Geometry check sheet. Reference: the model listing, model coordinates, mm. A direction names the side the tool comes from. Coordinates: 2 decimals unless noted, no trailing zeros. Loops run counter-clockwise (first coordinate to the right, second up) from the corner with the lowest first, then second, coordinate; pieces in that order, holes last.
from build123d import *
from OCP.BRepFilletAPI import BRepFilletAPI_MakeChamfer

# Parameters (mm, degrees)
BOSS_EXTRUDE1_DEPTH     = 5
CHAMFER1_SIZE           = 5
CHAMFER1_SIZE2          = 18.660254038
CUT_EXTRUDE1_DEPTH      = 10
CUT_EXTRUDE1_DEPTH_BACK = 10


with BuildPart() as part:
    # Sketch1 → Boss-Extrude1 (new body)
    with BuildSketch(Plane(origin=(0, 0, 0), x_dir=(1, 0, 0), z_dir=(0, 1, 0))):
        Polygon((-7.5, 40), (7.5, 40), (7.5, -40), (1, -40), (1, -35), (-1, -35), (-1, -40), (-7.5, -40), align=None)
        with BuildLine():
            Line((-2.5, -25.078773429), (-2.5, 9.921226571))
            ThreePointArc((-2.5, 9.921226571), (0, 12.421226571), (2.5, 9.921226571))
            Line((2.5, 9.921226571), (2.5, -25.078773429))
            ThreePointArc((2.5, -25.078773429), (0, -27.578773429), (-2.5, -25.078773429))
        make_face(mode=Mode.SUBTRACT)
    extrude(amount=BOSS_EXTRUDE1_DEPTH)

    # Chamfer1: one chamfer whose edges measure the first distance from different faces: ONE call of the kernel's chamfer builder (chamfer() names one face for all edges)
    chamfer1_edges_1 = [part.edges().sort_by_distance(p)[0] for p in [
        (-7.5, 2.5, 40),
    ]]
    chamfer1_side_1 = [part.faces().sort_by_distance(p)[0] for p in [
        (-4.25, 2.5, 40),
    ]]
    chamfer1_edges_2 = [part.edges().sort_by_distance(p)[0] for p in [
        (7.5, 2.5, 40),
    ]]
    chamfer1_side_2 = [part.faces().sort_by_distance(p)[0] for p in [
        (4.25, 2.5, 40),
    ]]
    chamfer1 = BRepFilletAPI_MakeChamfer(part.part.solid().wrapped)
    for e in chamfer1_edges_1:
        chamfer1.Add(CHAMFER1_SIZE, CHAMFER1_SIZE2, e.wrapped, chamfer1_side_1[0].wrapped)  # the first distance lies on this face
    for e in chamfer1_edges_2:
        chamfer1.Add(CHAMFER1_SIZE, CHAMFER1_SIZE2, e.wrapped, chamfer1_side_2[0].wrapped)  # the first distance lies on this face
    add(Compound.cast(chamfer1.Shape()), mode=Mode.REPLACE)

    # Sketch2 → Cut-Extrude1 (cut, two sides: drawn at the far end of the back side and taken through both)
    with BuildSketch(Plane(origin=(0, 0, 0), x_dir=(0, 0, -1), z_dir=(1, 0, 0)).offset(-CUT_EXTRUDE1_DEPTH_BACK)):
        Polygon((-42.19528089, 0.706295209), (-15.143740131, 5.709375865), (-42.19528089, 5.709375865), align=None)
    extrude(amount=CUT_EXTRUDE1_DEPTH + CUT_EXTRUDE1_DEPTH_BACK, mode=Mode.SUBTRACT)


solid = part.part
(1) Scan lines: L1, parallel to X at y = 0.85, z = 0; L2, parallel to X at y = 3, z = 25. Record each from-to range of solid material in increasing order.
Findings:
L1: x = -7.5 to -2.5, 2.5 to 7.5
L2: x = -6.52 to -2.5, 2.5 to 6.52
(2) Sectioned sample at B-B on x = 0. Record the cut outline in (y, z), and give its area (3 significant figures).
Findings:
outline: (0, -40) - (5, -40) - (5, -12.42) - (0, -12.42) - close; (0, 27.58) - (3.41, 27.58) - (2.04, 35) - (0, 35) - close
area: 158 mm2
(3) Sectioned sample at D-D on x = 5.25. Record the cut outline in (y, z).
Findings:
outline: (0, -40) - (5, -40) - (5, 18.98) - (3.01, 29.74) - (0, 29.74) - close
(4) Gauge pin test, flat ends, axial feed: pin 1 Ø1 at (x, y) = (0, 1) entering from +Z; pin 2 Ø0.6 at (y, z) = (1.5, 38.5) entering from -X; pin 3 Ø2 at (y, z) = (1, 37.5) entering from +X. Record the tip position at first contact, or that the pin passes through.
Findings:
pin 1: stops at z = 35
pin 2: stops at x = -2.98
pin 3: stops at x = 3.44
(5) Sectioned sample at A-A on z = -3. Record the cut outline in (x, y), and give its area (3 significant figures).
Findings:
outline: (-7.5, 0) - (-2.5, 0) - (-2.5, 5) - (-7.5, 5) - close; (2.5, 0) - (7.5, 0) - (7.5, 5) - (2.5, 5) - close
area: 50.0 mm2
(6) Sectioned sample at C-C on y = 2.75. Record the cut outline in (x, z).
Findings:
outline: (-7.5, -40) - (7.5, -40) - (7.5, 21.34) - (4.87, 31.15) - (-4.87, 31.15) - (-7.5, 21.34) - close; hole (-2.5, -9.92) arc R2.5 ccw to (2.5, -9.92) - (2.5, 25.08) arc R2.5 ccw to (-2.5, 25.08) - close
(7) Access from +Z, -Z, +X, -X, +Y, -Y to the whole of each face (thin tool, end or side, straight path). Record for faces 1 (the flat face through (-2.5, 2, 8)), 2 (the flat face through (3, 0, -9)), 3 (the flat face through (0, 1, 35)).
Findings:
face 1: +Y, -Y
face 2: +Z, -Z, +X, -X, -Y
face 3: +Z, +Y, -Y
(8) Draft check along X on faces 4 (the cylindrical face through (-0.05, 2.46, -12.42)), 5 (the flat face through (0, 2, -40)), 6 (the flat face through (7.5, 2, -10)), 7 (the cylindrical face through (0.05, 1.91, 27.58)). Enter one of: +X half, -X half, draft (parallel to the pull), parting line (faces both ways), or undercut.
Findings:
face 4: undercut
face 5: draft
face 6: +X half
face 7: undercut
